```python
from build123d import *

# Parameters (mm, degrees)
SKETCH_1_W           = 25
SKETCH_1_H           = 25
SKETCH_1_W_2         = 23
SKETCH_1_H_2         = 23
EXTRUDE_1_DEPTH      = 40
SKETCH_4_R           = 1.5
CUT_EXTRUDE_3_DEPTH  = 10
SKETCH_17_R          = 3.75
CUT_EXTRUDE_16_DEPTH = 1
CUT_EXTRUDE_17_REACH = 50.798
SKETCH_18_R          = 1.505


with BuildPart() as part:
    # 草图1 → 凸台-拉伸1 (new, symmetric)
    with BuildSketch(Plane.XY):
        Rectangle(SKETCH_1_W, SKETCH_1_H)
        Rectangle(SKETCH_1_W_2, SKETCH_1_H_2, mode=Mode.SUBTRACT)
    extrude(amount=EXTRUDE_1_DEPTH, both=True)

    # 草图4 → 切除-拉伸3 (cut)
    with BuildSketch(Plane.ZY.offset(-11.5)):
        with Locations(Location((25.05, -7.5, 0), (0, 0, 270))):
            Circle(SKETCH_4_R)
        with Locations(Location((25.05, 7.5, 0), (0, 0, 270))):
            Circle(SKETCH_4_R)
        with Locations(Location((9.05, 7.5, 0), (0, 0, 270))):
            Circle(SKETCH_4_R)
        with Locations(Location((9.05, -7.5, 0), (0, 0, 270))):
            Circle(SKETCH_4_R)
    extrude(amount=-CUT_EXTRUDE_3_DEPTH, mode=Mode.SUBTRACT)

    # 草图17 → 切除-拉伸16 (cut)
    with BuildSketch(Plane.ZY.offset(12.5)):
        with Locations(Location((25.05, 7.5, 0), (0, 0, 270))):
            Circle(SKETCH_17_R)
        with Locations(Location((9.05, 7.5, 0), (0, 0, 270))):
            Circle(SKETCH_17_R)
        with Locations(Location((25.05, -7.5, 0), (0, 0, 270))):
            Circle(SKETCH_17_R)
        with Locations(Location((9.05, -7.5, 0), (0, 0, 270))):
            Circle(SKETCH_17_R)
    extrude(amount=-CUT_EXTRUDE_16_DEPTH, mode=Mode.SUBTRACT)

    # 切除-拉伸17: up to this face of the body (flat: up to its plane)
    cut_extrude_17_end = Plane(part.part.faces().sort_by_distance((12.5, 0, -0.244495165))[0])
    # 草图18 → 切除-拉伸17 (cut, up to the picked face)
    with BuildSketch(Plane.ZY.offset(12.5), mode=Mode.PRIVATE) as cut_extrude_17_sk1:
        with Locations(Location((-36, 8.5, 0), (0, 0, 270))):
            Circle(SKETCH_18_R)
    cut_extrude_17_tool1 = split(extrude(cut_extrude_17_sk1.sketch, amount=-CUT_EXTRUDE_17_REACH, mode=Mode.PRIVATE), bisect_by=cut_extrude_17_end, keep=Keep.BOTH, mode=Mode.PRIVATE)
    # 草图18 → 切除-拉伸17 (cut, up to the picked face)
    with BuildSketch(Plane.ZY.offset(12.5), mode=Mode.PRIVATE) as cut_extrude_17_sk2:
        with Locations(Location((-14, 8.5, 0), (0, 0, 270))):
            Circle(SKETCH_18_R)
    cut_extrude_17_tool2 = split(extrude(cut_extrude_17_sk2.sketch, amount=-CUT_EXTRUDE_17_REACH, mode=Mode.PRIVATE), bisect_by=cut_extrude_17_end, keep=Keep.BOTH, mode=Mode.PRIVATE)
    # 草图18 → 切除-拉伸17 (cut, up to the picked face)
    with BuildSketch(Plane.ZY.offset(12.5), mode=Mode.PRIVATE) as cut_extrude_17_sk3:
        with Locations(Location((-14, -8.5, 0), (0, 0, 270))):
            Circle(SKETCH_18_R)
    cut_extrude_17_tool3 = split(extrude(cut_extrude_17_sk3.sketch, amount=-CUT_EXTRUDE_17_REACH, mode=Mode.PRIVATE), bisect_by=cut_extrude_17_end, keep=Keep.BOTH, mode=Mode.PRIVATE)
    # 草图18 → 切除-拉伸17 (cut, up to the picked face)
    with BuildSketch(Plane.ZY.offset(12.5), mode=Mode.PRIVATE) as cut_extrude_17_sk4:
        with Locations(Location((-36, -8.5, 0), (0, 0, 270))):
            Circle(SKETCH_18_R)
    cut_extrude_17_tool4 = split(extrude(cut_extrude_17_sk4.sketch, amount=-CUT_EXTRUDE_17_REACH, mode=Mode.PRIVATE), bisect_by=cut_extrude_17_end, keep=Keep.BOTH, mode=Mode.PRIVATE)
    add(cut_extrude_17_tool1.solids().sort_by(Axis((-12.5, 8.5, -36), (1, 0, 0)))[0], mode=Mode.SUBTRACT)
    add(cut_extrude_17_tool2.solids().sort_by(Axis((-12.5, 8.5, -14), (1, 0, 0)))[0], mode=Mode.SUBTRACT)
    add(cut_extrude_17_tool3.solids().sort_by(Axis((-12.5, -8.5, -14), (1, 0, 0)))[0], mode=Mode.SUBTRACT)
    add(cut_extrude_17_tool4.solids().sort_by(Axis((-12.5, -8.5, -36), (1, 0, 0)))[0], mode=Mode.SUBTRACT)


solid = part.part
```
Here's how the part is built. I have some questions about the finished solid (model axes, mm). A direction names the side the tool comes from. Give positions to 0.01 mm unless a question says otherwise; leave off trailing zeros. Order: outer loops, then holes, each group sorted by start corner. A loop starts at its lowest first (then second) coordinate and runs counter-clockwise, first axis right, second up. Notation, with made-up numbers: M 37,-7 L 92,-7 A12 ccw 92,7 Z; hole C -14,26.5 d8. An arc over 180 degrees is marked long. Use a Markdown table: item, result. Add a question column.
1. I need wall thicknesses on probe 1 along Y at (x, z) = (3, -31.5); probe 2 along Z at (x, y) = (12.2, 8.5) (3 decimals). Which ranges of each line are inside material? Lowest first, please. Write a range as from..to.
2. Suppose I cut it at B-B (x = -7.5). List the corners of the cut face in (y, z) for me, and give its area (3 significant figures).
3. On a 3-axis mill with a long thin cutter (end or side, diameter ignored), from which of +Z, -Z, +X, -X, +Y, -Y can I reach the whole of each face in a straight line? I mean faces 1 (the cylindrical face through (-12.007, -9.194, -37.335)), 2 (the flat face through (-11.5, 0, 1)), 3 (the cylindrical face through (-12.01, 8.31, 5.39)). Say none if no direction works.
4. If we mould it in two halves opening along X, with no side actions, what happens to faces 4 (the flat face through (-12.5, 0, 1)), 5 (the flat face through (0, 11.5, 1)), 6 (the cylindrical face through (-12.01, 7.69, -12.73)), 7 (the flat face through (12.5, 0, 1))? For each: +X half, -X half, draft (parallel to the pull), parting line (faces both ways), or undercut.
5. Suppose I cut it at C-C (y = 4.5). List the corners of the cut face in (x, z) for me.
6. For pin 1 Ø4 at (y, z) = (-8.5, -36) entering from -X; pin 2 Ø1.8 at (y, z) = (-7.5, 25.05) entering from +X; pin 3 Ø7 at (y, z) = (7.5, 25.05) entering from -X, each with a flat end and sliding along its axis, tell me the tip position at first contact or that it passes through.
7. Suppose I cut it at D-D (z = -21.5). List the corners of the cut face in (x, y) for me.
8. Suppose I cut it at A-A (z = 9.05). List the corners of the cut face in (x, y) for me.
Results list:
| question | item | result |
|---|---|---|
| 1 | probe 1 | y = -12.5..-11.5, 11.5..12.5 |
| 1 | probe 2 | z = -40..-37.505, -34.495..-15.505, -12.495..7.932, 10.168..23.932, 26.168..40 |
| 2 | outline | M -12.5,-40 L -11.5,-40 L -11.5,40 L -12.5,40 Z; M 11.5,-40 L 12.5,-40 L 12.5,40 L 11.5,40 Z |
| 2 | area | 160 mm² |
| 3 | face 1 | +X, -X |
| 3 | face 2 | +Z, -Z |
| 3 | face 3 | -X |
| 4 | face 4 | -X half |
| 4 | face 5 | undercut |
| 4 | face 6 | draft |
| 4 | face 7 | +X half |
| 5 | outline | M -12.5,-40 L -11.5,-40 L -11.5,6.8 L -12.5,6.8 Z; M -12.5,11.3 L -11.5,11.3 L -11.5,22.8 L -12.5,22.8 Z; M -12.5,27.3 L -11.5,27.3 L -11.5,40 L -12.5,40 Z; M 11.5,-40 L 12.5,-40 L 12.5,40 L 11.5,40 Z |
| 6 | pin 1 | stops at x = -12.5 |
| 6 | pin 2 | passes through |
| 6 | pin 3 | stops at x = 11.5 |
| 7 | outline | M -12.5,-12.5 L 12.5,-12.5 L 12.5,12.5 L -12.5,12.5 Z; hole M -11.5,-11.5 L 11.5,-11.5 L 11.5,11.5 L -11.5,11.5 Z |
| 8 | outline | M -12.5,-12.5 L 12.5,-12.5 L 12.5,-9 L 11.5,-9 L 11.5,-11.5 L -11.5,-11.5 L -11.5,-11.25 L -12.5,-11.25 Z; M -12.5,-3.75 L -11.5,-3.75 L -11.5,3.75 L -12.5,3.75 Z; M -12.5,11.25 L -11.5,11.25 L -11.5,11.5 L 11.5,11.5 L 11.5,9 L 12.5,9 L 12.5,12.5 L -12.5,12.5 Z; M 11.5,-6 L 12.5,-6 L 12.5,6 L 11.5,6 Z |
